Job drawing, mm, ordinate dimensions from the low corner. One solid piece. A direction names the side the tool comes from. Give positions to 0.01 mm unless a question says otherwise; leave off trailing zeros. Loops run counter-clockwise (first coordinate to the right, second up) from the corner with the lowest first, then second, coordinate; pieces in that order, holes last. Notation, with made-up numbers: (-28, 41.25) - (-17, 41.25) arc R10 ccw to (-17, 48.25) - close; hole circle Ø9 at (85, -23.5). An arc over 180 degrees is marked (long way). Use a Markdown table: item, result.
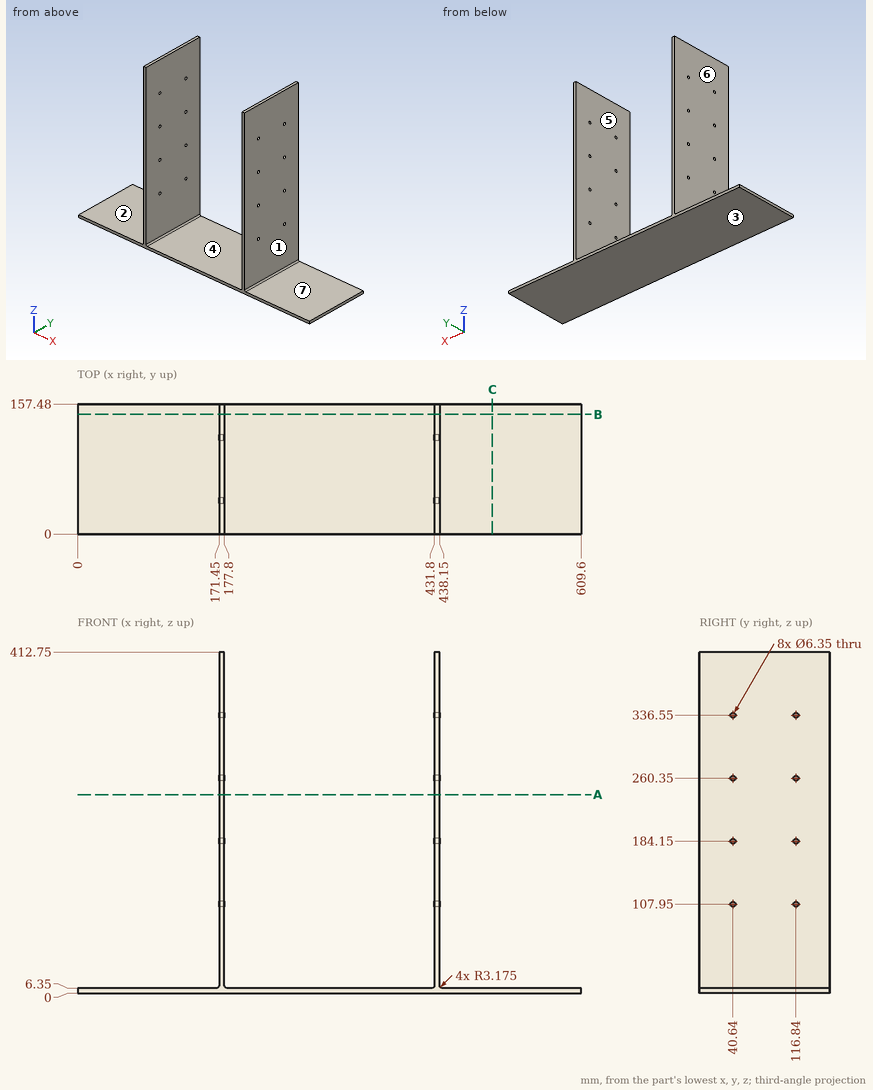
(1) Drill centre lines: probe 1 along Z at (x, y) = (175.5, 40.64) (3 decimals); probe 2 along Y at (x, z) = (434, 184); probe 3 along X at (y, z) = (18, 186.5). Where is each one in solid material? Low to high. Write a range as [from, to].
Computed:
| item | result |
|---|---|
| probe 1 | [0, 104.775], [111.125, 180.975], [187.325, 257.175], [263.525, 333.375], [339.725, 412.75] |
| probe 2 | [0, 37.47], [43.81, 113.67], [120.01, 157.48] |
| probe 3 | [171.45, 177.8], [431.8, 438.15] |
(2) Slice it at B-B, the plane y = 145. Write the cut outline in (x, z) (3 decimals).
Computed:
| item | result |
|---|---|
| outline | (0, 0) - (609.6, 0) - (609.6, 6.35) - (441.325, 6.35) arc R3.175 cw to (438.15, 9.525) - (438.15, 412.75) - (431.8, 412.75) - (431.8, 9.525) arc R3.175 cw to (428.625, 6.35) - (180.975, 6.35) arc R3.175 cw to (177.8, 9.525) - (177.8, 412.75) - (171.45, 412.75) - (171.45, 9.525) arc R3.175 cw to (168.275, 6.35) - (0, 6.35) - close |
(3) Slice it at C-C, the plane x = 502. Write the cut outline in (y, z), plus the area to 4 significant figures.
Computed:
| item | result |
|---|---|
| outline | (0, 0) - (157.48, 0) - (157.48, 6.35) - (0, 6.35) - close |
| area | 1,000 mm² |
(4) Pin check, flat tips, straight feed: P1, Ø12, axis at y = 141.5, z = 337, coming from the +X side; P2, Ø1, axis at x = 139.5, y = 105.5, coming from the +Z side; P3, Ø8.5, axis at y = 116.84, z = 107.95, coming from the +X side; P4, Ø5.5, axis at y = 116.84, z = 260.35, coming from the -X side. Stop position of each tip, or through.
Computed:
| item | result |
|---|---|
| P1 | x = 438.15 |
| P2 | z = 6.35 |
| P3 | x = 438.15 |
| P4 | through |
(5) Slice it at A-A, the plane z = 240.5. Write the cut outline in (x, y), plus the area to 3 significant figures.
Computed:
| item | result |
|---|---|
| outline | (171.45, 0) - (177.8, 0) - (177.8, 157.48) - (171.45, 157.48) - close; (431.8, 0) - (438.15, 0) - (438.15, 157.48) - (431.8, 157.48) - close |
| area | 2,000 mm² |
(6) Mould opens along X. For the marked faces 5, 6 and 7 say: pulls with the +X half, pulls with the -X half, needs draft (parallel to the pull), parting line crosses it, or undercut.
Computed:
| item | result |
|---|---|
| face 5 | undercut |
| face 6 | pulls with the -X half |
| face 7 | needs draft |
(7) 3-axis set-ups, long thin cutter, end or side, ignore diameter. For the marked faces 1, 2, 3 and 4: which of +Z, -Z, +X, -X, +Y, -Y reach the whole face in a straight line?
Computed:
| item | result |
|---|---|
| face 1 | +Z, +X, +Y, -Y |
| face 2 | +Z, -X, +Y, -Y |
| face 3 | -Z, +X, -X, +Y, -Y |
| face 4 | +Z, +Y, -Y |
